The model under review builds one solid part; all positions refer to its coordinate system, in mm. A direction names the side the tool comes from. Coordinates: 2 decimals unless noted, no trailing zeros. Write each loop counter-clockwise with the first axis right and the second up, starting at its lowest first coordinate (ties: lowest second). Pieces come first, ordered by that corner, then holes.
1) Machinability: for faces 1 (the cylindrical face through (5.703, 1.521, -73.986)), 2 (the flat face through (60, 2, -3)), which of the approach directions +Z, -Z, +X, -X, +Y, -Y give a long, thin tool a straight path to every point of the face, cutting with its end or side? Answer none if there is none.
2) Mouldability with a two-part tool opening along X and no side actions: class faces 3 (the cylindrical face through (74.297, 1.521, -6.014)), 4 (the cylindrical face through (54.9, 1.5, -14.1)), 5 (the flat face through (40, 1, 0)) as released by +X, released by -X, zero draft, split by the parting line, or undercut.
3) For P1, Ø1.8, axis at x = 4, z = -48, coming from the -Y side (3 decimals); P2, Ø1.5, axis at y = 1.5, z = -7.5, coming from the +X side, all flat-tipped, find the tip position at first contact; note any pin that passes through.
4) Add section D-D, the plane x = 4. State the section outline as (y, z) points.
5) Add section A-A, the plane z = -48. State the section outline as (x, y) points, then the cut area to 3 significant figures.
6) Add section B-B, the plane y = 1.8. Give the number of separate pieces and of enclosed holes in the cut face, then the cut area to 3 significant figures.
7) For line 1 (Z direction, x = 60, y = 0.85); line 2 (X direction, y = 0.3, z = -48); line 3 (X direction, y = 0.9, z = -5), list the stretches that pass through material, from the lowest coordinate up.
8) Add section C-C, the plane x = 50. State the section outline as (y, z) points.
from build123d import *

# Parameters (mm, degrees)
SKETCH3_W           = 80
SKETCH3_H           = 80
BOSS_EXTRUDE1_DEPTH = 3
FILLET3_R           = 20
FILLET4_R           = 20
FILLET5_R           = 20
FILLET6_R           = 20
SKETCH12_R          = 1.5
CUT_EXTRUDE6_DEPTH  = 3
SKETCH13_R          = 1.5
CUT_EXTRUDE7_DEPTH  = 3
SKETCH14_R          = 1.5
CUT_EXTRUDE8_DEPTH  = 10
SKETCH15_W          = 14
SKETCH15_H          = 8.5
CUT_EXTRUDE9_DEPTH  = 10


with BuildPart() as part:
    # Sketch3 → Boss-Extrude1 (new body)
    with BuildSketch(Plane(origin=(0, 0, 0), x_dir=(1, 0, 0), z_dir=(0, 1, 0))):
        with Locations((40, 40)):
            Rectangle(SKETCH3_W, SKETCH3_H)
    extrude(amount=BOSS_EXTRUDE1_DEPTH)

    # Fillet3
    fillet3_edges = [part.edges().sort_by_distance(p)[0] for p in [
        (0, 1.5, -80),
    ]]
    fillet(fillet3_edges, radius=FILLET3_R)

    # Fillet4
    fillet4_edges = [part.edges().sort_by_distance(p)[0] for p in [
        (80, 1.5, -80),
    ]]
    fillet(fillet4_edges, radius=FILLET4_R)

    # Fillet5
    fillet5_edges = [part.edges().sort_by_distance(p)[0] for p in [
        (80, 1.5, 0),
    ]]
    fillet(fillet5_edges, radius=FILLET5_R)

    # Fillet6
    fillet6_edges = [part.edges().sort_by_distance(p)[0] for p in [
        (0, 1.5, 0),
    ]]
    fillet(fillet6_edges, radius=FILLET6_R)

    # Sketch12 → Cut-Extrude6 (cut)
    with BuildSketch(Plane(origin=(0, 3, 0), x_dir=(1, 0, 0), z_dir=(0, 1, 0))):
        with Locations((30, 5)):
            Circle(SKETCH12_R)
        with Locations((50, 5)):
            Circle(SKETCH12_R)
    extrude(amount=-CUT_EXTRUDE6_DEPTH, mode=Mode.SUBTRACT)

    # Sketch13 → Cut-Extrude7 (cut)
    with BuildSketch(Plane(origin=(0, 3, 0), x_dir=(1, 0, 0), z_dir=(0, 1, 0))):
        with Locations((20, 70)):
            Circle(SKETCH13_R)
        with Locations((60, 70)):
            Circle(SKETCH13_R)
    extrude(amount=-CUT_EXTRUDE7_DEPTH, mode=Mode.SUBTRACT)

    # Sketch14 → Cut-Extrude8 (cut)
    with BuildSketch(Plane(origin=(0, 3, 0), x_dir=(1, 0, 0), z_dir=(0, 1, 0))):
        with Locations((4, 20.1)):
            Circle(SKETCH14_R)
        with Locations((4, 48)):
            Circle(SKETCH14_R)
        with Locations((54.8, 63.2)):
            Circle(SKETCH14_R)
        with Locations((56.1, 15)):
            Circle(SKETCH14_R)
    extrude(amount=-CUT_EXTRUDE8_DEPTH, mode=Mode.SUBTRACT)

    # Sketch15 → Cut-Extrude9 (cut)
    with BuildSketch(Plane(origin=(0, 3, 0), x_dir=(1, 0, 0), z_dir=(0, 1, 0))):
        with Locations((60, 7.25)):
            Rectangle(SKETCH15_W, SKETCH15_H)
    extrude(amount=-CUT_EXTRUDE9_DEPTH, mode=Mode.SUBTRACT)


solid = part.part
Geometry results:
1. face 1: -Z, -X, +Y, -Y
1. face 2: +Y, -Y
2. face 3: released by +X
2. face 4: undercut
2. face 5: zero draft
3. P1: passes through
3. P2: stops at x = 76.18
4. outline: (0, -72) - (3, -72) - (3, -49.5) - (0, -49.5) - close; (0, -46.5) - (3, -46.5) - (3, -21.6) - (0, -21.6) - close; (0, -18.6) - (3, -18.6) - (3, -8) - (0, -8) - close
5. outline: (0, 0) - (2.5, 0) - (2.5, 3) - (0, 3) - close; (5.5, 0) - (80, 0) - (80, 3) - (5.5, 3) - close
5. area: 231 mm2
6. separate pieces: 1
6. enclosed holes: 9
6. area: 5,880 mm2
7. line 1: z = -80 to -71.5, -68.5 to -11.5, -3 to 0
7. line 2: x = 0 to 2.5, 5.5 to 80
7. line 3: x = 6.77 to 28.5, 31.5 to 48.5, 51.5 to 53, 67 to 73.23
8. outline: (0, -80) - (3, -80) - (3, -6.5) - (0, -6.5) - close; (0, -3.5) - (3, -3.5) - (3, 0) - (0, 0) - close
